from build123d import *

# Parameters (mm, degrees)
SKETCH_R     = 2.5
PAD_DEPTH    = 5
SKETCH002_R  = 1.2
POCKET_DEPTH = 25.001


with BuildPart() as part:
    # Sketch → Pad (new body)
    with BuildSketch(Plane.XY):
        with BuildLine():
            ThreePointArc((0, 3.5), (-3.5, 0), (0, -3.5))
            Line((57.98, -3.5), (0, -3.5))
            ThreePointArc((57.98, -3.5), (61.48, 0), (57.98, 3.5))
            Line((0, 3.5), (57.98, 3.5))
        make_face()
        Circle(SKETCH_R, mode=Mode.SUBTRACT)
        with Locations((57.98, 0)):
            Circle(SKETCH_R, mode=Mode.SUBTRACT)
    extrude(amount=PAD_DEPTH)

    # Sketch002 → Pocket (cut, through all)
    with BuildSketch(Plane.XY.offset(25)):
        with Locations((20, 0)):
            Circle(SKETCH002_R)
        with Locations((38, 0)):
            Circle(SKETCH002_R)
    extrude(amount=-POCKET_DEPTH, mode=Mode.SUBTRACT)


solid = part.part
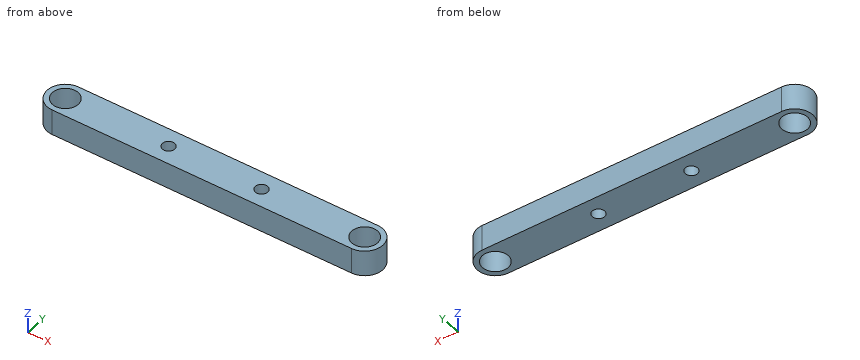
Check sheet for the modelled part. Datum: model origin and axes. Units: mm. Coordinates: 2 decimals unless noted, no trailing zeros. Loops run counter-clockwise (first coordinate to the right, second up) from the corner with the lowest first, then second, coordinate; pieces in that order, holes last. Notation, with made-up numbers: (-35, 83.25) -> (-2, 83.25) arc R27 ccw to (-2, 101.25) -> close; hole circle Ø11 at (29.5, -34). An arc over 180 degrees is marked (long way). Answer in a Markdown table with one row per item.
1. Sectioned sample at C-C, the plane z = 1.85. Record the boundary of the cut face in (x, y), then the cut area to 3 significant figures.
Check values:
| item | result |
|---|---|
| outline | (0, -3.5) -> (57.98, -3.5) arc R3.5 ccw to (57.98, 3.5) -> (0, 3.5) arc R3.5 ccw to start; hole circle Ø5 at (0, 0); hole circle Ø2.4 at (20, 0); hole circle Ø2.4 at (38, 0); hole circle Ø5 at (57.98, 0) |
| area | 396 mm2 |
2. Material ranges on line 1 along Y through (x, z) = (57.98, 1.9); line 2 along Y through (x, z) = (20, 1.1); line 3 along X through (y, z) = (-1, 1.3), recorded low to high. Write a range as [from, to].
Check values:
| item | result |
|---|---|
| line 1 | y = [-3.5, -2.5], [2.5, 3.5] |
| line 2 | y = [-3.5, -1.2], [1.2, 3.5] |
| line 3 | x = [-3.35, -2.29], [2.29, 19.34], [20.66, 37.34], [38.66, 55.69], [60.27, 61.33] |
3. Sectioned sample at A-A, the plane y = 0. Record the boundary of the cut face in (x, z).
Check values:
| item | result |
|---|---|
| outline | (-3.5, 0) -> (-2.5, 0) -> (-2.5, 5) -> (-3.5, 5) -> close; (2.5, 0) -> (18.8, 0) -> (18.8, 5) -> (2.5, 5) -> close; (21.2, 0) -> (36.8, 0) -> (36.8, 5) -> (21.2, 5) -> close; (39.2, 0) -> (55.48, 0) -> (55.48, 5) -> (39.2, 5) -> close; (60.48, 0) -> (61.48, 0) -> (61.48, 5) -> (60.48, 5) -> close |
4. Sectioned sample at B-B, the plane x = 38. Record the boundary of the cut face in (y, z).
Check values:
| item | result |
|---|---|
| outline | (-3.5, 0) -> (-1.2, 0) -> (-1.2, 5) -> (-3.5, 5) -> close; (1.2, 0) -> (3.5, 0) -> (3.5, 5) -> (1.2, 5) -> close |
